Can you work these out from the model? Positions are in its coordinate system, mm. Give positions to 0.01 mm unless a question says otherwise; leave off trailing zeros. Write each loop counter-clockwise with the first axis right and the second up, starting at its lowest first coordinate (ties: lowest second). Pieces come first, ordered by that corner, then holes.
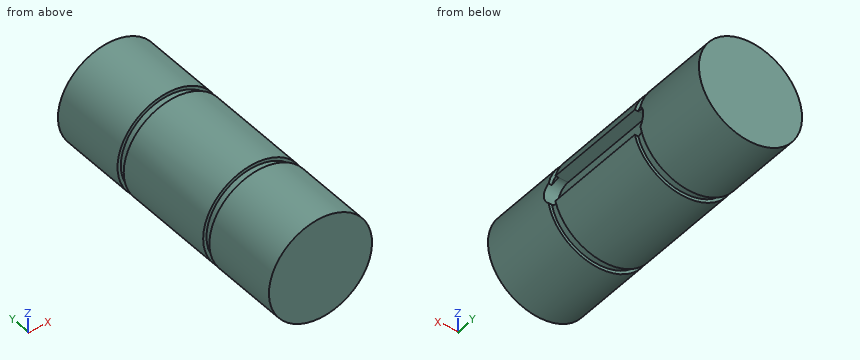
```python
from build123d import *

# Parameters (mm, degrees)
SKETCH1_R           = 2.5
BOSS_EXTRUDE1_DEPTH = 13.28
SKETCH2_W           = 6.44702982
SKETCH2_H           = 0.39
SKETCH3_W           = 6.610697995
SKETCH3_H           = 0.39
CUT_EXTRUDE1_DEPTH  = 0.7


with BuildPart() as part:
    # Sketch1 → Boss-Extrude1 (new body)
    with BuildSketch(Plane(origin=(0, 0, 0), x_dir=(1, 0, 0), z_dir=(0, 1, 0))):
        with Locations(Location((0, 0, 0), (0, 0, 90))):
            Circle(SKETCH1_R)
    extrude(amount=BOSS_EXTRUDE1_DEPTH)

    # Sketch2 → Cut-Revolve1 (revolve, cut)
    with BuildSketch(Plane(origin=(0, 0, 0), x_dir=(0, 0, -1), z_dir=(1, 0, 0)), mode=Mode.PRIVATE) as cut_revolve1_sk:
        with Locations((-5.56351491, 9.335)):
            Rectangle(SKETCH2_W, SKETCH2_H)
    revolve(cut_revolve1_sk.sketch.rotate(Axis((0, 10.194505394, 0), (0, -1, 0)), 180), axis=Axis((0, 10.194505394, 0), (0, -1, 0)), mode=Mode.SUBTRACT)

    # Sketch3 → Cut-Revolve2 (revolve, cut)
    with BuildSketch(Plane(origin=(0, 0, 0), x_dir=(0, 0, -1), z_dir=(1, 0, 0)), mode=Mode.PRIVATE) as cut_revolve2_sk:
        with Locations((-5.645348998, 3.945)):
            Rectangle(SKETCH3_W, SKETCH3_H)
    revolve(cut_revolve2_sk.sketch.rotate(Axis((0, 6.07806317, 0), (0, -1, 0)), 180), axis=Axis((0, 6.07806317, 0), (0, -1, 0)), mode=Mode.SUBTRACT)

    # Sketch4 → Cut-Extrude1 (cut)
    with BuildSketch(Plane(origin=(2.5, 0, 0), x_dir=(0, 0, -1), z_dir=(1, 0, 0))):
        with BuildLine():
            Line((0.625, 9.14), (0.625, 4.14))
            ThreePointArc((0.625, 4.14), (0, 3.515), (-0.625, 4.14))
            Line((-0.625, 4.14), (-0.625, 9.14))
            ThreePointArc((-0.625, 9.14), (0, 9.765), (0.625, 9.14))
        make_face()
    extrude(amount=-CUT_EXTRUDE1_DEPTH, mode=Mode.SUBTRACT)


solid = part.part
```
1) Please list where these lines run through material, in increasing order: L1, parallel to X at y = 8.75, z = 0.05; L2, parallel to X at y = 5.5, z = -0.7; L3, parallel to Z at x = -1.95, y = 7.5.
Values follow:
L1: x = -2.5 to 1.8
L2: x = -2.4 to 2.4
L3: z = -1.56 to 1.56
2) Suppose I cut it at B-B on y = 2.5. Write out the boundary of the cut face in (x, z).
Values follow:
outline: circle Ø5 at (0, 0)
3) Suppose I cut it at C-C on x = -2.2. Write out the boundary of the cut face in (y, z), plus the area to 3 significant figures.
Values follow:
outline: (0, -1.19) - (3.75, -1.19) - (3.75, -0.8) - (4.14, -0.8) - (4.14, -1.19) - (9.14, -1.19) - (9.14, -0.8) - (9.53, -0.8) - (9.53, -1.19) - (13.28, -1.19) - (13.28, 1.19) - (9.53, 1.19) - (9.53, 0.8) - (9.14, 0.8) - (9.14, 1.19) - (4.14, 1.19) - (4.14, 0.8) - (3.75, 0.8) - (3.75, 1.19) - (0, 1.19) - close
area: 30.9 mm2
4) Suppose I cut it at A-A on z = 0. Write out the boundary of the cut face in (x, y) (3 decimals).
Values follow:
outline: (-2.5, 0) - (2.5, 0) - (2.5, 3.515) - (1.8, 3.515) - (1.8, 9.765) - (2.5, 9.765) - (2.5, 13.28) - (-2.5, 13.28) - (-2.5, 9.53) - (-2.34, 9.53) - (-2.34, 9.14) - (-2.5, 9.14) - (-2.5, 4.14) - (-2.34, 4.14) - (-2.34, 3.75) - (-2.5, 3.75) - close
5) For pin 1 Ø2 at (y, z) = (3.5, 1.5) entering from +X; pin 2 Ø1 at (y, z) = (6, 0) entering from +X; pin 3 Ø1 at (x, z) = (0, 0) entering from -Y, each with a flat end and sliding along its axis, tell me the tip position at first contact or that it passes through.
Values follow:
pin 1: stops at x = 2.45
pin 2: stops at x = 1.8
pin 3: stops at y = 0
6) Suppose I cut it at D-D on z = 1.9. Write out the boundary of the cut face in (x, y).
Values follow:
outline: (-1.62, 0) - (1.62, 0) - (1.62, 3.75) - (1.37, 3.75) - (1.37, 4.14) - (1.62, 4.14) - (1.62, 9.14) - (1.37, 9.14) - (1.37, 9.53) - (1.62, 9.53) - (1.62, 13.28) - (-1.62, 13.28) - (-1.62, 9.53) - (-1.37, 9.53) - (-1.37, 9.14) - (-1.62, 9.14) - (-1.62, 4.14) - (-1.37, 4.14) - (-1.37, 3.75) - (-1.62, 3.75) - close
